Study the drawing (mm; zero at the part's minimum x, y, z) and answer. A direction names the side the tool comes from. Round coordinates to 2 decimals unless told otherwise and drop trailing zeros. Loops run counter-clockwise (first coordinate to the right, second up) from the corner with the lowest first, then second, coordinate; pieces in that order, holes last. Notation, with made-up numbers: (18.5, -22) -> (68.5, -22) arc R16 ccw to (68.5, 0) -> close; hole circle Ø5 at (62, 12). An arc over 180 degrees is marked (long way). Use one line per item in the form item = value.
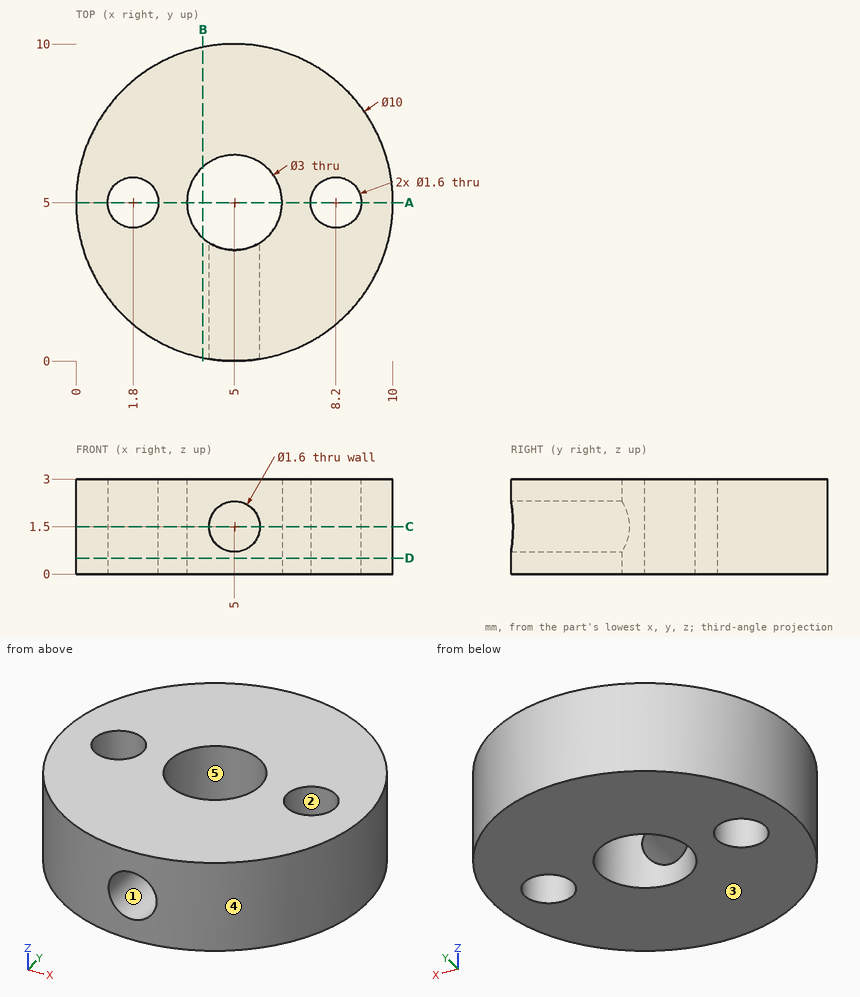
(1) Find section A-A, the plane y = 5. Write down the section's boundary in (x, z).
Completed:
outline = (0, 0) -> (1, 0) -> (1, 3) -> (0, 3) -> close; (2.6, 0) -> (3.5, 0) -> (3.5, 3) -> (2.6, 3) -> close; (6.5, 0) -> (7.4, 0) -> (7.4, 3) -> (6.5, 3) -> close; (9, 0) -> (10, 0) -> (10, 3) -> (9, 3) -> close
(2) For the marked faces 1 and 2, determine the directions among +Z, -Z, +X, -X, +Y, -Y from which every point of the face is accessible in a straight line to the end or side of a thin tool.
Completed:
face_1 = -Y
face_2 = +Z, -Z
(3) Consider L1, parallel to X at y = 5.5, z = 2.55; L2, parallel to Y at x = 8.75, z = 2.35; L3, parallel to Y at x = 2, z = 2.2. Determine where each line is inside the solid, lowest interval first.
Completed:
L1 = 0.03 to 1.18, 2.42 to 3.59, 6.41 to 7.58, 8.82 to 9.97
L2 = 1.69 to 4.42, 5.58 to 8.31
L3 = 1 to 4.23, 5.77 to 9
(4) Find section C-C, the plane z = 1.5. Write down the section's boundary in (x, y), then the cut area to 3 significant figures.
Completed:
outline = (4.2, 0.06) -> (4.2, 3.73) arc R1.5 cw (long way) to (5.8, 3.73) -> (5.8, 0.06) arc R5 ccw (long way) to start; hole circle Ø1.6 at (1.8, 5); hole circle Ø1.6 at (8.2, 5)
area = 61.8 mm2
(5) Given P1, Ø1.5, axis at y = 2, z = 1, coming from the -X side, flat-ended and moving along its own axis, determine where the tip first touches the part or whether it passes through.
Completed:
P1 = 0.53
(6) For a pull along X with two mould halves and no side action, classify the marked faces 3, 4 and 5 as +X half, -X half, draft (parallel to the pull), parting line (faces both ways), or undercut.
Completed:
face_3 = draft
face_4 = parting line
face_5 = undercut
(7) Find section B-B, the plane x = 4. Write down the section's boundary in (y, z), then the cut area to 3 significant figures.
Completed:
outline = (0.1, 0) -> (3.88, 0) -> (3.88, 3) -> (0.1, 3) -> close; (6.12, 0) -> (9.9, 0) -> (9.9, 3) -> (6.12, 3) -> close
area = 22.7 mm2
(8) Find section D-D, the plane z = 0.5. Write down the section's boundary in (x, y), then the cut area to 4 significant figures.
Completed:
outline = circle Ø10 at (5, 5); hole circle Ø1.6 at (1.8, 5); hole circle Ø3 at (5, 5); hole circle Ø1.6 at (8.2, 5)
area = 67.45 mm2
